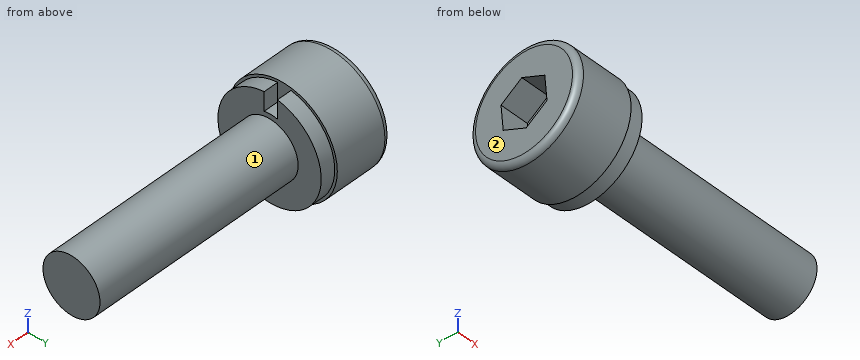
from build123d import *

# Parameters (mm, degrees)
CUT_EXTRUDE_1_DEPTH = 1
FILLET_1_R          = 0.2
CUT_EXTRUDE_2_DEPTH = 0.51


with BuildPart() as part:
    # 草图1 → 旋转1 (revolve)
    with BuildSketch(Plane.XY):
        Polygon((0, 0), (0, 1.9), (2, 1.9), (2, 1.81), (2.51, 1.81), (2.51, 1), (10, 1), (10, 0), align=None)
    revolve(axis=Axis((0, 0, 0), (1, 0, 0)))

    # 草图2 → 切除-拉伸1 (cut)
    with BuildSketch(Plane.ZY):
        Polygon((0.510545523, -0.727926234), (0.885675372, 0.078182276), (0.375129849, 0.80610851), (-0.510545523, 0.727926234), (-0.885675372, -0.078182276), (-0.375129849, -0.80610851), align=None)
    extrude(amount=-CUT_EXTRUDE_1_DEPTH, mode=Mode.SUBTRACT)

    # 圆角1
    fillet_1_edges = [part.edges().sort_by_distance(p)[0] for p in [
        (0, -1.9, 0),
    ]]
    fillet(fillet_1_edges, radius=FILLET_1_R)

    # 草图3 → 切除-拉伸2 (cut)
    with BuildSketch(Plane(origin=(2.51, 0, 0), x_dir=(0, 0, -1), z_dir=(1, 0, 0))):
        with BuildLine():
            Line((-1.138940095, 0.275804569), (-1.788863281, 0.275804569))
            ThreePointArc((-1.788863281, 0.275804569), (-1.809465078, 0.044001494), (-1.800154668, -0.188528969))
            Line((-1.800154668, -0.188528969), (-1.143106206, -0.188528969))
            ThreePointArc((-1.143106206, -0.188528969), (-1.168348286, 0.043882968), (-1.138940095, 0.275804569))
        make_face()
    extrude(amount=-CUT_EXTRUDE_2_DEPTH, mode=Mode.SUBTRACT)


solid = part.part
Work out the finished part from the listing and answer in its coordinate system (mm). Face numbers are marked on the shaded views. A direction names the side the tool comes from. Round coordinates to 2 decimals unless told otherwise and drop trailing zeros. Write each loop counter-clockwise with the first axis right and the second up, starting at its lowest first coordinate (ties: lowest second). Pieces come first, ordered by that corner, then holes. Notation, with made-up numbers: (7.25, 66) -> (13.25, 66) arc R23 ccw to (13.25, 100) -> close; hole circle Ø4 at (13.5, -21.5). An arc over 180 degrees is marked (long way). Answer as CSV lines item,"result". Start each with the question number.
(1) The part is cut by section A-A, the plane x = 2.25. Give the vertices of the cut face in (y, z), then the cut area to 3 significant figures.
(2) Find the intervals of material crossed by probe 1 along X at (y, z) = (-1.65, 0.15); probe 2 along X at (y, z) = (0.3, -0.1); probe 3 along Y at (x, z) = (9.5, 0.55), in increasing order.
(3) The part is cut by section B-B, the plane x = 5.5. Give the vertices of the cut face in (y, z).
(4) Each of these flat-tipped pins is pushed along its axis until it touches: pin 1 (0.6 mm diameter, centred on x = 2.5, z = 1.5, fed in from +Y) (3 decimals); pin 2 (1.5 mm diameter, centred on x = 6.5, y = 0.5, fed in from -Z); pin 3 (0.6 mm diameter, centred on x = 2.5, z = 1.5, fed in from -Y) (3 decimals). Where does it stop, or does it pass through?
(5) A tool of negligible diameter and unlimited length cuts with its end or side. For the marked faces 1 and 2, from which of +Z, -Z, +X, -X, +Y, -Y can it reach the whole face along a straight path? Write none if from no direction.
Output values:
1,outline,"(-0.19, 1.14) -> (-0.19, 1.8) arc R1.81 ccw (long way) to (0.28, 1.79) -> (0.28, 1.14) arc R1 ccw to start"
1,area,"9.99 mm²"
2,probe 1,"x = 0 to 2.51"
2,probe 2,"x = 1 to 10"
2,probe 3,"y = -0.84 to 0.84"
3,outline,"circle Ø2 at (0, 0)"
4,pin 1,"stops at y = 1.355"
4,pin 2,"stops at z = -1"
4,pin 3,"stops at y = -1.355"
5,face 1,"+X"
5,face 2,"+Z, -Z, -X, +Y, -Y"
